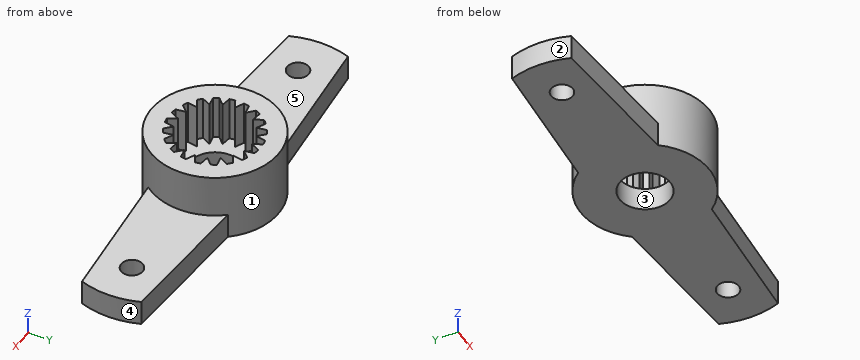
from build123d import *

# Parameters (mm, degrees)
SKETCH2_R           = 3.55
BOSS_EXTRUDE1_DEPTH = 3.8
BOSS_EXTRUDE2_DEPTH = 1.4
SKETCH5_R           = 2.549999919
CUT_EXTRUDE1_DEPTH  = 2.5
BOSS_EXTRUDE3_DEPTH = 2.5
SKETCH6_R           = 1.4
CUT_EXTRUDE2_DEPTH  = 12.745554295
SKETCH7_R           = 0.6
CUT_EXTRUDE3_DEPTH  = 12.724676785


with BuildPart() as part:
    # Sketch2 → Boss-Extrude1 (new body)
    with BuildSketch(Plane.XY):
        Circle(SKETCH2_R)
    extrude(amount=-BOSS_EXTRUDE1_DEPTH)

    # Sketch4 → Boss-Extrude2 (add)
    with BuildSketch(Plane.XY.offset(-2.4)):
        with BuildLine():
            Line((2.776387215, 2.212277889), (10.622617722, 1.649999976))
            ThreePointArc((10.622617722, 1.649999976), (10.913548722, 0), (10.622617722, -1.649999976))
            Line((10.622617722, -1.649999976), (2.776387215, -2.212277889))
            ThreePointArc((2.776387215, -2.212277889), (3.549999952, 0), (2.776387215, 2.212277889))
        make_face()
    boss_extrude2 = extrude(amount=-BOSS_EXTRUDE2_DEPTH)

    # Sketch5 → Cut-Extrude1 (cut)
    with BuildSketch(Plane.XY):
        Circle(SKETCH5_R)
    extrude(amount=-CUT_EXTRUDE1_DEPTH, mode=Mode.SUBTRACT)

    # Sketch3 → Boss-Extrude3 (add)
    with BuildSketch(Plane.XY):
        with BuildLine():
            Line((-0.244697916, 2.538232164), (0, 2.049999952))
            Line((0, 2.049999952), (0.244697916, 2.538232164))
            ThreePointArc((0.244697916, 2.538232164), (0, 2.549999919), (-0.244697916, 2.538232164))
        make_face()
        with BuildLine():
            Line((0.551635326, 2.489618054), (0.633484824, 1.949665813))
            Line((0.633484824, 1.949665813), (1.017078422, 2.338386424))
            ThreePointArc((1.017078422, 2.338386424), (0.787993311, 2.42519404), (0.551635326, 2.489618054))
        make_face()
        with BuildLine():
            Line((1.29397066, 2.197302783), (1.204959739, 1.6584848))
            Line((1.204959739, 1.6584848), (1.689900206, 1.90964313))
            ThreePointArc((1.689900206, 1.90964313), (1.498852346, 2.06299327), (1.29397066, 2.197302783))
        make_face()
        with BuildLine():
            Line((1.90964313, 1.689900206), (1.6584848, 1.204959739))
            Line((1.6584848, 1.204959739), (2.197302783, 1.29397066))
            ThreePointArc((2.197302783, 1.29397066), (2.06299327, 1.498852346), (1.90964313, 1.689900206))
        make_face()
        with BuildLine():
            Line((2.338386424, 1.017078422), (1.949665813, 0.633484824))
            Line((1.949665813, 0.633484824), (2.489618054, 0.551635326))
            ThreePointArc((2.489618054, 0.551635326), (2.42519404, 0.787993311), (2.338386424, 1.017078422))
        make_face()
        with BuildLine():
            Line((2.538232164, 0.244697916), (2.049999952, 0))
            Line((2.049999952, 0), (2.538232164, -0.244697916))
            ThreePointArc((2.538232164, -0.244697916), (2.549999919, 0), (2.538232164, 0.244697916))
        make_face()
        with BuildLine():
            Line((2.489618054, -0.551635326), (1.949665813, -0.633484824))
            Line((1.949665813, -0.633484824), (2.338386424, -1.017078422))
            ThreePointArc((2.338386424, -1.017078422), (2.42519404, -0.787993311), (2.489618054, -0.551635326))
        make_face()
        with BuildLine():
            Line((2.197302783, -1.29397066), (1.6584848, -1.204959739))
            Line((1.6584848, -1.204959739), (1.90964313, -1.689900206))
            ThreePointArc((1.90964313, -1.689900206), (2.06299327, -1.498852346), (2.197302783, -1.29397066))
        make_face()
        with BuildLine():
            Line((1.689900206, -1.90964313), (1.204959739, -1.6584848))
            Line((1.204959739, -1.6584848), (1.29397066, -2.197302783))
            ThreePointArc((1.29397066, -2.197302783), (1.498852346, -2.06299327), (1.689900206, -1.90964313))
        make_face()
        with BuildLine():
            Line((1.017078422, -2.338386424), (0.633484824, -1.949665813))
            Line((0.633484824, -1.949665813), (0.551635326, -2.489618054))
            ThreePointArc((0.551635326, -2.489618054), (0.787993311, -2.42519404), (1.017078422, -2.338386424))
        make_face()
        with BuildLine():
            Line((0.244697916, -2.538232164), (0, -2.049999952))
            Line((0, -2.049999952), (-0.244697916, -2.538232164))
            ThreePointArc((-0.244697916, -2.538232164), (0, -2.549999919), (0.244697916, -2.538232164))
        make_face()
        with BuildLine():
            Line((-0.551635326, -2.489618054), (-0.633484824, -1.949665813))
            Line((-0.633484824, -1.949665813), (-1.017078422, -2.338386424))
            ThreePointArc((-1.017078422, -2.338386424), (-0.787993311, -2.42519404), (-0.551635326, -2.489618054))
        make_face()
        with BuildLine():
            Line((-1.29397066, -2.197302783), (-1.204959739, -1.6584848))
            Line((-1.204959739, -1.6584848), (-1.689900206, -1.90964313))
            ThreePointArc((-1.689900206, -1.90964313), (-1.498852346, -2.06299327), (-1.29397066, -2.197302783))
        make_face()
        with BuildLine():
            Line((-1.90964313, -1.689900206), (-1.6584848, -1.204959739))
            Line((-1.6584848, -1.204959739), (-2.197302783, -1.29397066))
            ThreePointArc((-2.197302783, -1.29397066), (-2.06299327, -1.498852346), (-1.90964313, -1.689900206))
        make_face()
        with BuildLine():
            Line((-2.338386424, -1.017078422), (-1.949665813, -0.633484824))
            Line((-1.949665813, -0.633484824), (-2.489618054, -0.551635326))
            ThreePointArc((-2.489618054, -0.551635326), (-2.42519404, -0.787993311), (-2.338386424, -1.017078422))
        make_face()
        with BuildLine():
            Line((-2.538232164, -0.244697916), (-2.049999952, 0))
            Line((-2.049999952, 0), (-2.538232164, 0.244697916))
            ThreePointArc((-2.538232164, 0.244697916), (-2.549999919, 0), (-2.538232164, -0.244697916))
        make_face()
        with BuildLine():
            Line((-2.489618054, 0.551635326), (-1.949665813, 0.633484824))
            Line((-1.949665813, 0.633484824), (-2.338386424, 1.017078422))
            ThreePointArc((-2.338386424, 1.017078422), (-2.42519404, 0.787993311), (-2.489618054, 0.551635326))
        make_face()
        with BuildLine():
            Line((-2.197302783, 1.29397066), (-1.6584848, 1.204959739))
            Line((-1.6584848, 1.204959739), (-1.90964313, 1.689900206))
            ThreePointArc((-1.90964313, 1.689900206), (-2.06299327, 1.498852346), (-2.197302783, 1.29397066))
        make_face()
        with BuildLine():
            Line((-1.689900206, 1.90964313), (-1.204959739, 1.6584848))
            Line((-1.204959739, 1.6584848), (-1.29397066, 2.197302783))
            ThreePointArc((-1.29397066, 2.197302783), (-1.498852346, 2.06299327), (-1.689900206, 1.90964313))
        make_face()
        with BuildLine():
            Line((-1.017078422, 2.338386424), (-0.633484824, 1.949665813))
            Line((-0.633484824, 1.949665813), (-0.551635326, 2.489618054))
            ThreePointArc((-0.551635326, 2.489618054), (-0.787993311, 2.42519404), (-1.017078422, 2.338386424))
        make_face()
    extrude(amount=-BOSS_EXTRUDE3_DEPTH)

    # Sketch6 → Cut-Extrude2 (cut, through all)
    with BuildSketch(Plane.XY.offset(-2.5)):
        Circle(SKETCH6_R)
    extrude(amount=-CUT_EXTRUDE2_DEPTH, mode=Mode.SUBTRACT)

    # Sketch7 → Cut-Extrude3 (cut, through all)
    with BuildSketch(Plane.XY.offset(-2.4)):
        with Locations((8.5405208, 0)):
            Circle(SKETCH7_R)
    cut_extrude3 = extrude(amount=-CUT_EXTRUDE3_DEPTH, mode=Mode.SUBTRACT)

    # Mirror1: Boss-Extrude2 across plane
    add(boss_extrude2.mirror(Plane(origin=(0, 0, 0), x_dir=(0, 0, 1), z_dir=(1, 0, 0))))

    # Mirror2: Cut-Extrude3 across plane
    add(cut_extrude3.mirror(Plane(origin=(0, 0, 0), x_dir=(0, 0, 1), z_dir=(1, 0, 0))), mode=Mode.SUBTRACT)


solid = part.part
Check sheet for the modelled part. Datum: model origin and axes. Units: mm. Face numbers are marked on the shaded views. A direction names the side the tool comes from. Coordinates: 2 decimals unless noted, no trailing zeros. Write each loop counter-clockwise with the first axis right and the second up, starting at its lowest first coordinate (ties: lowest second). Pieces come first, ordered by that corner, then holes.
Item 1: Access from +Z, -Z, +X, -X, +Y, -Y to the whole of each face (thin tool, end or side, straight path). Record for the marked faces 1 and 2.
Numbers:
face 1: +Z
face 2: +Z, -Z, -X
Item 2: Scan lines: probe 1 along Z at (x, y) = (-10, 0); probe 2 along X at (y, z) = (0.25, -2.8); probe 3 along X at (y, z) = (-1.75, -2.3). Record each from-to range of solid material in increasing order.
Numbers:
probe 1: z = -3.8 to -2.4
probe 2: x = -10.91 to -9.09, -8 to -1.38, 1.38 to 8, 9.09 to 10.91
probe 3: x = -3.09 to -1.85, -1.38 to -1.22, 1.22 to 1.38, 1.85 to 3.09
Item 3: Cross-section at C-C on y = 3. Record the boundary of the cut face in (x, z), then the cut area to 3 significant figures.
Numbers:
outline: (-1.9, -3.8) - (1.9, -3.8) - (1.9, 0) - (-1.9, 0) - close
area: 14.4 mm2
Item 4: Depth check by flat-ended pin: pin 1 Ø1 at (x, y) = (-5, 1) entering from +Z; pin 2 Ø1 at (x, z) = (-5.5, -1) entering from +Y; pin 3 Ø3.5 at (x, y) = (0, 0) entering from -Z; pin 4 Ø1 at (y, z) = (-1, -3) entering from +X. Enter the tip coordinate at first touch or a pass-through.
Numbers:
pin 1: stops at z = -2.4
pin 2: passes through
pin 3: stops at z = -3.8
pin 4: stops at x = 10.89
Item 5: Mould release check, pull along Y, two halves, no side actions. Record for the marked faces 3, 4 and 5: released by +Y, released by -Y, zero draft, split by the parting line, or undercut.
Numbers:
face 3: undercut
face 4: split by the parting line
face 5: zero draft
Item 6: Cross-section at A-A on z = -3.5. Record the boundary of the cut face in (x, y), then the cut area to 3 significant figures.
Numbers:
outline: (-10.62, -1.65) - (-2.78, -2.21) arc R3.55 ccw to (2.78, -2.21) - (10.62, -1.65) arc R4.82 ccw to (10.62, 1.65) - (2.78, 2.21) arc R3.55 ccw to (-2.78, 2.21) - (-10.62, 1.65) arc R4.82 ccw to start; hole circle Ø1.2 at (-8.54, 0); hole circle Ø2.8 at (0, 0); hole circle Ø1.2 at (8.54, 0)
area: 88.4 mm2
Item 7: Cross-section at B-B on x = 5.75. Record the boundary of the cut face in (y, z), then the cut area to 3 significant figures.
Numbers:
outline: (-2, -3.8) - (2, -3.8) - (2, -2.4) - (-2, -2.4) - close
area: 5.60 mm2
